Check sheet for the modelled part. Datum: model origin and axes. Units: mm. A direction names the side the tool comes from. Give positions to 0.01 mm unless a question says otherwise; leave off trailing zeros. Loops run counter-clockwise (first coordinate to the right, second up) from the corner with the lowest first, then second, coordinate; pieces in that order, holes last. Notation, with made-up numbers: M 85.25,25.25 L 137.25,25.25 A25 ccw 137.25,58.25 Z; hole C 77.25,55 d1. An arc over 180 degrees is marked long. Write each question's results on one line, items separated by ' | '. Start each with the question number.
1. Material ranges on line 1 along X through (y, z) = (17, 0); line 2 along Z through (x, y) = (0, 26.5); line 3 along Z through (x, y) = (88.5, 18), recorded low to high.
2. Draft check along X on faces 1 (the flat face through (49, 20, 15)), 2 (the flat face through (61, 22, -10)), 3 (the cylindrical face through (115, 20, 0)), 4 (the cylindrical face through (110, 22, 0)). Enter one of: pulls with the +X half, pulls with the -X half, needs draft (parallel to the pull), parting line crosses it, or undercut.
3. Tool access check on faces 5 (the flat face through (0, 4, 0)), 6 (the flat face through (34.6, 40, -10.2)). Record the directions out of +Z, -Z, +X, -X, +Y, -Y that give a thin tool (end or side, any length) a straight path to the whole face; none if there is none.
4. Sectioned sample at B-B on z = 0. Record the cut outline in (x, y).
5. Sectioned sample at A-A on y = 15. Record the cut outline in (x, z), and give its area (3 significant figures).
6. Sectioned sample at C-C on x = 28. Record the cut outline in (y, z).
7. Go/stop test with flat-tipped pins: pin 1 (8 mm diameter, centred on y = 5, z = 2, fed in from +X); pin 2 (1 mm diameter, centred on x = 85, z = 0.5, fed in from +Y); pin 3 (10 mm diameter, centred on y = 21.5, z = -8.5, fed in from -X). Record where each tip stops, or that it passes through.
```python
from build123d import *

# Parameters (mm, degrees)
SKETCH1_R           = 6
BOSS_EXTRUDE1_DEPTH = 40
SKETCH1_2_R         = 6
BOSS_EXTRUDE2_DEPTH = 4


with BuildPart() as part:
    # Sketch1 → Boss-Extrude1 (new body)
    with BuildSketch(Plane(origin=(0, 0, 0), x_dir=(1, 0, 0), z_dir=(0, 1, 0))):
        with BuildLine():
            Line((0, -15), (100, -15))
            ThreePointArc((100, -15), (115, 0), (100, 15))
            Line((100, 15), (0, 15))
            ThreePointArc((0, 15), (-15, 0), (0, -15))
        make_face()
        Circle(SKETCH1_R, mode=Mode.SUBTRACT)
        with BuildLine():
            Line((23, 10), (100, 10))
            ThreePointArc((100, 10), (110, 0), (100, -10))
            Line((100, -10), (23, -10))
            ThreePointArc((23, -10), (13, 0), (23, 10))
        make_face(mode=Mode.SUBTRACT)
    extrude(amount=BOSS_EXTRUDE1_DEPTH)

    # Sketch1<2> → Boss-Extrude2 (add)
    with BuildSketch(Plane(origin=(0, 0, 0), x_dir=(1, 0, 0), z_dir=(0, 1, 0))):
        with BuildLine():
            Line((100, 10), (23, 10))
            ThreePointArc((23, 10), (13, 0), (23, -10))
            Line((23, -10), (100, -10))
            ThreePointArc((100, -10), (110, 0), (100, 10))
        make_face()
        Circle(SKETCH1_2_R)
    extrude(amount=BOSS_EXTRUDE2_DEPTH)


solid = part.part
```
Output values:
1) line 1: -15 to -6, 6 to 13, 110 to 115 | line 2: -15 to -6, 6 to 15 | line 3: -15 to -10, 10 to 15
2) face 1: needs draft | face 2: undercut | face 3: pulls with the +X half | face 4: undercut
3) face 5: +Y | face 6: +Z, -Z, +X, -X, +Y
4) outline: M -15,0 L 115,0 L 115,40 L 110,40 L 110,4 L 13,4 L 13,40 L 6,40 L 6,4 L -6,4 L -6,40 L -15,40 Z
5) outline: M 0,-15 L 100,-15 A15 ccw 100,15 L 0,15 A15 ccw Z; hole C 0,0 d12; hole M 23,-10 L 100,-10 A10 ccw 100,10 L 23,10 A10 ccw Z | area: 1,740 mm2
6) outline: M 0,-15 L 40,-15 L 40,-10 L 4,-10 L 4,10 L 40,10 L 40,15 L 0,15 Z
7) pin 1: x = 115 | pin 2: y = 4 | pin 3: x = -14.59
